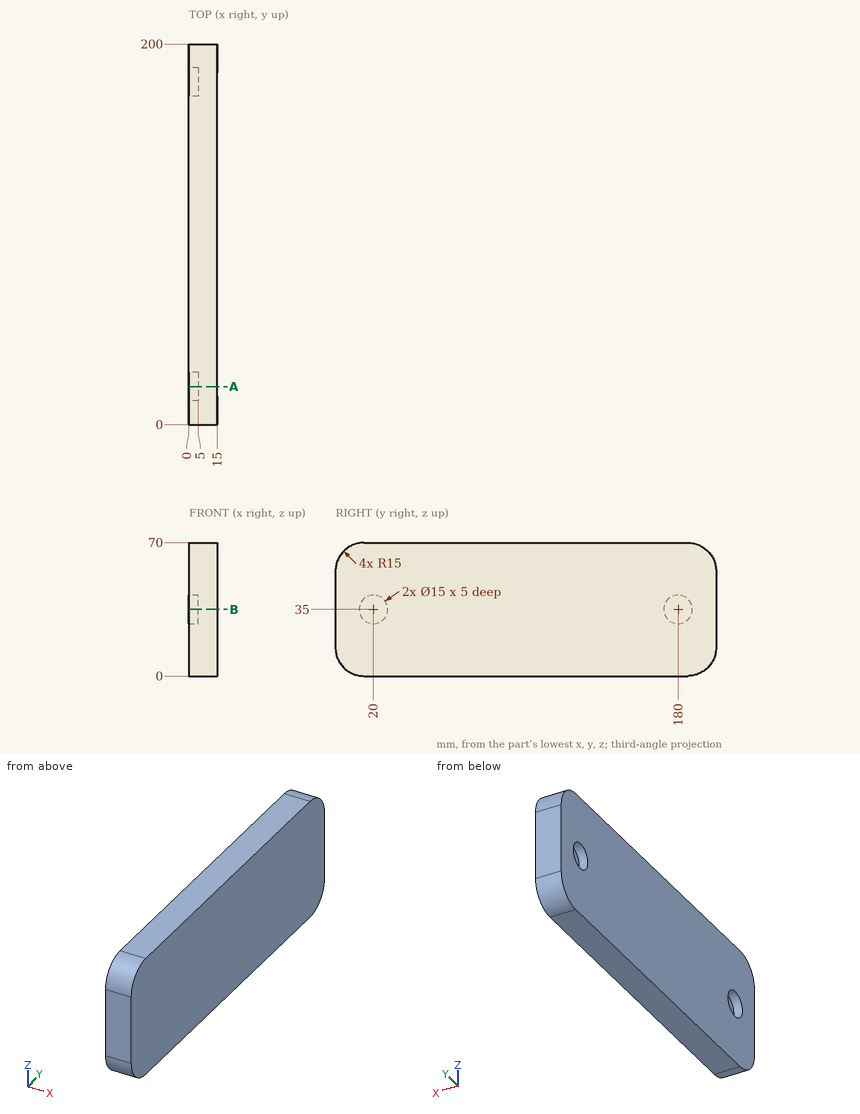
Check sheet for the drawn part. Datum: minimum x, y, z corner. Units: mm. Round coordinates to 2 decimals unless told otherwise and drop trailing zeros. Write each loop counter-clockwise with the first axis right and the second up, starting at its lowest first coordinate (ties: lowest second). Pieces come first, ordered by that corner, then holes. Notation, with made-up numbers: (38, -6) -> (66, -6) arc R14 ccw to (66, 16) -> close; hole circle Ø1 at (-9.5, -5.5). An arc over 180 degrees is marked (long way). One line per item, written item: value. Start each with the question number.
(1) Cross-section at B-B, the plane z = 35. Record the cut outline in (x, y), and give its area (3 significant figures).
(2) Go/stop test with a flat-tipped pin: pin 1 Ø4.5 at (y, z) = (17, 36) entering from -X. Record where the tip stops, or that it passes through.
(3) Scan lines: line 1 (Y direction, x = 2.5, z = 35); line 2 (X direction, y = 183, z = 29.5); line 3 (Y direction, x = 7.25, z = 5.5). Record each from-to range of solid material in increasing order. Write a range as [from, to].
(4) Cross-section at A-A, the plane y = 20. Record the cut outline in (x, z).
Answer:
1. outline: (0, 0) -> (15, 0) -> (15, 200) -> (0, 200) -> (0, 187.5) -> (5, 187.5) -> (5, 172.5) -> (0, 172.5) -> (0, 27.5) -> (5, 27.5) -> (5, 12.5) -> (0, 12.5) -> close
1. area: 2,850 mm²
2. pin 1: x = 5
3. line 1: [0, 12.5], [27.5, 172.5], [187.5, 200]
3. line 2: [5, 15]
3. line 3: [3.39, 196.61]
4. outline: (0, 0) -> (15, 0) -> (15, 70) -> (0, 70) -> (0, 42.5) -> (5, 42.5) -> (5, 27.5) -> (0, 27.5) -> close
